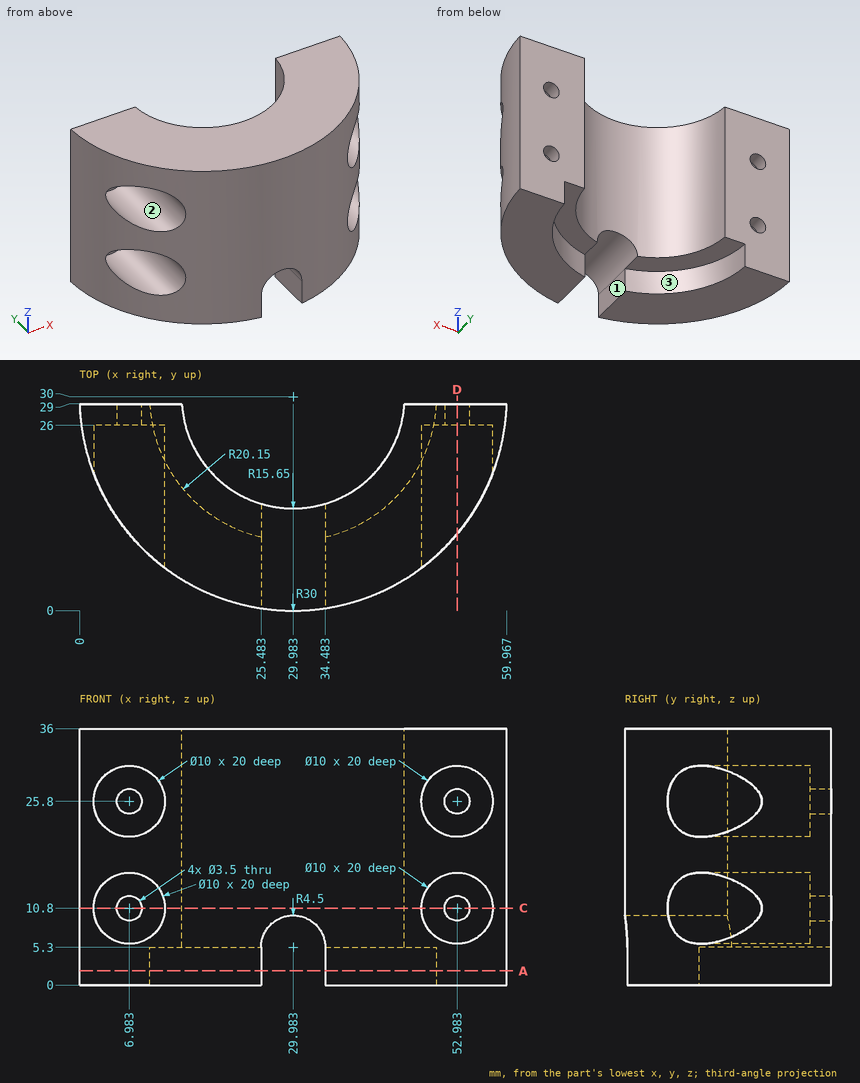
Verification items for this drawing (mm, ordinates from the low corner). A direction names the side the tool comes from. Coordinates: 2 decimals unless noted, no trailing zeros. Write each loop counter-clockwise with the first axis right and the second up, starting at its lowest first coordinate (ties: lowest second). Pieces come first, ordered by that corner, then holes. Notation, with made-up numbers: (72, 19.25) -> (93, 19.25) arc R8 ccw to (93, 26.25) -> close; hole circle Ø6 at (79.25, 0.5). An arc over 180 degrees is marked (long way). One line per item, written item: value. Start each with the question number.
Q1. Cross-section at C-C on z = 10.8. State how many separate pieces and enclosed holes the cut face has.
Q2. Cross-section at A-A on z = 2. Enter the section's corners in (x, y).
Q3. Access from +Z, -Z, +X, -X, +Y, -Y to the whole of each face (thin tool, end or side, straight path). Record for the marked faces 1, 2 and 3.
Q4. Go/stop test with flat-tipped pins: P1, Ø13, axis at x = 6.98, z = 25.8, coming from the -Y side; P2, Ø1.5, axis at x = 48.5, z = 9, coming from the -Y side; P3, Ø4, axis at x = 19, z = 27, coming from the -Y side. Record where each tip stops, or that it passes through.
Q5. Cross-section at D-D on x = 53. Enter the section's corners in (y, z).
Q6. Thickness scan on L1, parallel to Y at x = 30.5, z = 16 (1 decimal); L2, parallel to Z at x = 5, y = 21.25; L3, parallel to Z at x = 8, y = 25 (1 decimal). Record the ranges inside material, lowest first. Write a range as from..to.
Checked values:
1. separate pieces: 3
1. enclosed holes: 0
2. outline: (0, 29) arc R30 ccw to (25.48, 0.34) -> (25.48, 10.36) arc R20.15 cw to (9.86, 29) -> close; (34.48, 0.34) arc R30 ccw to (59.97, 29) -> (50.11, 29) arc R20.15 cw to (34.48, 10.36) -> close
3. face 1: -Z, +Y, -Y
3. face 2: -Y
3. face 3: -Z, +Y
4. P1: stops at y = 4.95
4. P2: stops at y = 5.83
4. P3: stops at y = 1.38
5. outline: (10.76, 0) -> (29, 0) -> (29, 9.05) -> (26, 9.05) -> (26, 5.8) -> (10.76, 5.8) -> close; (10.76, 15.8) -> (26, 15.8) -> (26, 12.55) -> (29, 12.55) -> (29, 24.05) -> (26, 24.05) -> (26, 20.8) -> (10.76, 20.8) -> close; (10.76, 30.8) -> (26, 30.8) -> (26, 27.55) -> (29, 27.55) -> (29, 36) -> (10.76, 36) -> close
6. L1: y = 0..14.4
6. L2: z = 0..6.21, 15.39..21.21, 30.39..36
6. L3: z = 0..5.9, 15.7..20.9, 30.7..36
